Check sheet for the modelled part. Datum: model origin and axes. Units: mm. A direction names the side the tool comes from. Give positions to 0.01 mm unless a question says otherwise; leave off trailing zeros. Order: outer loops, then holes, each group sorted by start corner. A loop starts at its lowest first (then second) coordinate and runs counter-clockwise, first axis right, second up.
Autodesk Inventor part; units mm, degrees
ref_plane "YZ Plane" through (0, 0, 0) normal (1, 0, 0) x (0, 1, 0)
ref_plane "XZ Plane" through (0, 0, 0) normal (0, 1, 0) x (-1, 0, 0)
ref_plane "XY Plane" through (0, 0, 0) normal (0, 0, 1) x (1, 0, 0)
sketch "Sketch1" plane through (0, 0, 0) normal (0, 0, 1) x (1, 0, 0)
  point P0 (0, 0)
sketch "Sketch2" plane through (0, 0, 0) normal (1, 0, 0) x (0, 1, 0)
  circle A0 centre (0, 0) radius 15
  circle A1 centre (0, -150) radius 15
  dimension "d0" = 30
  dimension "d1" = 30
  dimension "d2" = 150
  dimension "d3" = 0
extrude "Extrusion1" add sketch "Sketch2" along normal blind 125
sketch "Sketch3" plane through (0, 0, 0) normal (0, 0, 1) x (1, 0, 0)
  line L0 (125, -15) -> (125, 15)
  line L1 (0, 15) -> (0, -15)
  line L2 (0, 15) -> (125, 15)
  line L3 (0, -15) -> (125, -15)
  line L4 (125, 3) -> (0, 3)
  line L5 (0, 3) -> (0, -3)
  line L6 (0, -3) -> (125, -3)
  line L7 (125, -3) -> (125, 3)
  point P0 (0, 0)
  dimension "d10" = 3
  dimension "d11" = 3
extrude "Extrusion2" add sketch "Sketch3" against normal blind 150 contours L6 L1 L4 L0
sketch "Sketch4" plane through (0, -3, -14.6969) normal (0, -1, 0) x (1, 0, 0)
  point P0 (0, 14.6969)
sketch "Sketch5" plane through (0, 0, 0) normal (0, 1, 0) x (-1, 0, 0)
  line L0 (-125, -14.6969) -> (0, -14.6969)
  line L1 (-125, -14.6969) -> (-125, -135.3031)
  line L2 (0, -135.3031) -> (-125, -135.3031)
  line L3 (0, -14.6969) -> (0, -135.3031)
  line L4 (0, -14.6969) -> (-125, -14.6969)
  line L5 (-125, -14.6969) -> (-125, -14.6969)
  line L6 (-125, -14.6969) -> (0, -14.6969)
  line L7 (0, -14.6969) -> (0, -14.6969)
  line L8 (0, 15) -> (-125, 15)
  line L9 (0, -165) -> (-125, -165)
  circle A0 centre (-62.5, -75) radius 5
  point P0 (0, 0)
  dimension "d18" = 10
  dimension "d19" = 90
  dimension "d20" = 62.5
extrude "Extrusion3" cut sketch "Sketch5" along normal mid plane 6 contours A0
properties part number "EE_Base-Rod-Rev1"
1) Section check C-C, the plane z = -131.5. Record the cut outline in (x, y), then the cut area to 3 significant figures.
Recorded:
outline: (0, -3) - (125, -3) - (125, 3) - (0, 3) - close
area: 750 mm2
2) Section check A-A, the plane x = 62.5. Record the cut outline in (y, z).
Recorded:
outline: (-3, -135.3) arc R15 ccw (long way) to (3, -135.3) - (3, -80) - (-3, -80) - close; (-3, -70) - (3, -70) - (3, -14.7) arc R15 ccw (long way) to (-3, -14.7) - close
3) Section check B-B, the plane z = -75. Record the cut outline in (x, y), then the cut area to 3 significant figures.
Recorded:
outline: (0, -3) - (57.5, -3) - (57.5, 3) - (0, 3) - close; (67.5, -3) - (125, -3) - (125, 3) - (67.5, 3) - close
area: 690 mm2
4) Draft check along Z on faces 4 (the face through (0, 0, -81)), 5 (the face through (63.58, 0.04, -79.88)). Enter one of: +Z half, -Z half, draft (parallel to the pull), parting line (faces both ways), or undercut.
Recorded:
face 4: draft
face 5: undercut
5) Set-up check for faces 1 (the face through (63, 3, -88)), 2 (the face through (61.625, -0.617, 14.987)), 3 (the face through (62, -3, -88)): record each of +Z, -Z, +X, -X, +Y, -Y from which the full face is reachable in a straight line by a thin tool's end or side.
Recorded:
face 1: +X, -X, +Y
face 2: +X, -X
face 3: +X, -X, -Y
6) Material ranges on L1, parallel to Z at x = 62.5, y = -0.95; L2, parallel to Y at x = 60, z = -117; L3, parallel to Z at x = 14.5, y = -9.5, recorded low to high.
Recorded:
L1: z = -164.97 to -80, -70 to 14.97
L2: y = -3 to 3
L3: z = -161.61 to -138.39, -11.61 to 11.61
7) Depth check by flat-ended pin: pin 1 Ø3 at (x, z) = (50.5, -143.5) entering from -Y; pin 2 Ø1 at (x, y) = (81.5, 12) entering from -Z; pin 3 Ø10 at (x, z) = (87, -72.5) entering from +Y. Enter the tip coordinate at first touch or a pass-through.
Recorded:
pin 1: stops at y = -14.14
pin 2: stops at z = -159.63
pin 3: stops at y = 3
